from build123d import *

# Parameters (mm, degrees)
SKETCH1_W               = 484
SKETCH1_H               = 539
BASE_FLANGE1_DEPTH      = 1.89738
M6_CLEARANCE_HOLE1_D    = 6.6
CUT_EXTRUDE1_DEPTH      = 363.212437736
CUT_EXTRUDE1_DEPTH_BACK = 363.212437736


# Sheet-metal steps are written as plain solids
with BuildPart() as part:
    # Sketch1 → Base-Flange1 (new body)
    with BuildSketch(Plane.XY):
        Rectangle(SKETCH1_W, SKETCH1_H)
        with BuildLine():
            Line((136, -21.080107302), (136, -173.919892698))
            ThreePointArc((136, -173.919892698), (0, -253.5), (-136, -173.919892698))
            Line((-136, -173.919892698), (-136, -21.080107302))
            ThreePointArc((-136, -21.080107302), (0, 58.5), (136, -21.080107302))
        make_face(mode=Mode.SUBTRACT)
    extrude(amount=-BASE_FLANGE1_DEPTH)

    # M6 Clearance Hole1 (through all)
    with Locations(Plane(origin=(0, 0, -1.89738), x_dir=(-1, 0, 0), z_dir=(0, 0, -1))):
        with Locations((-226, 230), (226, 230), (226, -230), (-226, -230), (-226, 50), (226, 50)):
            Hole(M6_CLEARANCE_HOLE1_D / 2)

    # Sketch21 → Cut-Extrude1 (cut, two sides: drawn at the far end of the back side and taken through both)
    with BuildSketch(Plane.XY.offset(-CUT_EXTRUDE1_DEPTH_BACK)):
        with BuildLine():
            Line((-234, -218.5), (-234, -231.5))
            ThreePointArc((-234, -231.5), (-236.343145751, -237.156854249), (-242, -239.5))
            Line((-242, -239.5), (-242, -210.5))
            ThreePointArc((-242, -210.5), (-236.343145751, -212.843145751), (-234, -218.5))
        make_face()
    extrude(amount=CUT_EXTRUDE1_DEPTH + CUT_EXTRUDE1_DEPTH_BACK, mode=Mode.SUBTRACT)


solid = part.part
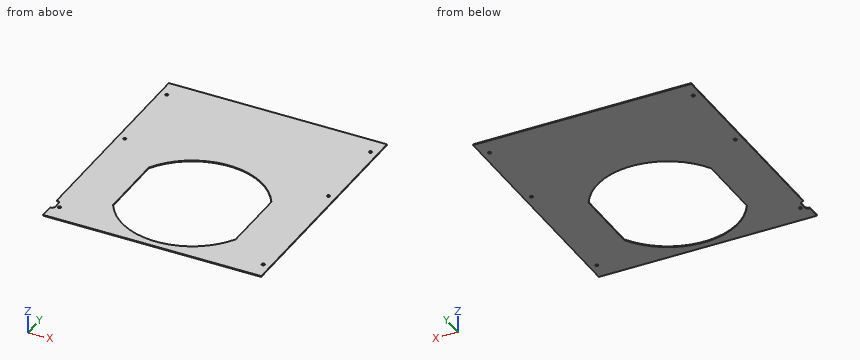
Work out the finished part from the listing and answer in its coordinate system (mm). Give positions to 0.01 mm unless a question says otherwise; leave off trailing zeros. Loops run counter-clockwise (first coordinate to the right, second up) from the corner with the lowest first, then second, coordinate; pieces in that order, holes last. Notation, with made-up numbers: (-9, -14) - (3, -14) arc R24 ccw to (3, 11) - close; hole circle Ø8 at (1, -35.75). An arc over 180 degrees is marked (long way). Answer in a Markdown table with one row per item. Add a question column.
Q1. The part is cut by section C-C (x = -66). Determine the outline of the cut face in (y, z), and give its area (3 significant figures).
Q2. The part is cut by section A-A (y = -105). Determine the outline of the cut face in (x, z).
Q3. The part is cut by section B-B (z = -1.2). Determine the outline of the cut face in (x, y).
Q4. Consider line 1 along Y through (x, z) = (-226, -0.4); line 2 along X through (y, z) = (230, -1.15); line 3 along X through (y, z) = (-168.5, -0.4). Determine where each line is inside the solid, lowest interval first.
Solution:
| question | item | result |
|---|---|---|
| 1 | outline | (-269.5, -1.9) - (-238.85, -1.9) - (-238.85, 0) - (-269.5, 0) - close; (43.85, -1.9) - (269.5, -1.9) - (269.5, 0) - (43.85, 0) - close |
| 1 | area | 486 mm² |
| 2 | outline | (-242, -1.9) - (-136, -1.9) - (-136, 0) - (-242, 0) - close; (136, -1.9) - (242, -1.9) - (242, 0) - (136, 0) - close |
| 3 | outline | (-242, -269.5) - (242, -269.5) - (242, 269.5) - (-242, 269.5) - (-242, -210.5) arc R8 cw to (-234, -218.5) - (-234, -231.5) arc R8 cw to (-242, -239.5) - close; hole circle Ø6.6 at (-226, -230); hole circle Ø6.6 at (-226, 50); hole circle Ø6.6 at (-226, 230); hole (-136, -173.92) arc R156 ccw to (136, -173.92) - (136, -21.08) arc R156 ccw to (-136, -21.08) - close; hole circle Ø6.6 at (226, -230); hole circle Ø6.6 at (226, 50); hole circle Ø6.6 at (226, 230) |
| 4 | line 1 | y = -269.5 to -233.3, -226.7 to 46.7, 53.3 to 226.7, 233.3 to 269.5 |
| 4 | line 2 | x = -242 to -229.3, -222.7 to 222.7, 229.3 to 242 |
| 4 | line 3 | x = -242 to -136, 136 to 242 |
